Verification items for the finished model (mm, model axes). A direction names the side the tool comes from. Give positions to 0.01 mm unless a question says otherwise; leave off trailing zeros. Order: outer loops, then holes, each group sorted by start corner. A loop starts at its lowest first (then second) coordinate and runs counter-clockwise, first axis right, second up. Notation, with made-up numbers: M 5,-11 L 31,-11 A24 cw 31,12 Z; hole C 53,44.25 d7. An arc over 180 degrees is marked long. Answer as a JSON object with one key per item and string values.
```python
from build123d import *

# Parameters (mm, degrees)
F0_W      = 90
F0_H      = 90
F1_DEPTH  = 90
F2_W      = 30
F2_H      = 30
F3_DEPTH  = 30
F4_W      = 30
F4_H      = 30
F5_DEPTH  = 30
F6_W      = 30
F6_H      = 30
F7_DEPTH  = 30
F8_W      = 30
F8_H      = 30
F9_DEPTH  = 30
F10_W     = 30
F10_H     = 30
F11_DEPTH = 30
F12_W     = 30
F12_H     = 30
F13_DEPTH = 30


with BuildPart() as f1:
    # F0 (on Top) → F1 (new body)
    with BuildSketch(Plane.XY):
        Rectangle(F0_W, F0_H)
    extrude(amount=F1_DEPTH)

    # F2 (on face) → F3 (join)
    with BuildSketch(Plane(origin=(0, 0, 0), x_dir=(1, 0, 0), z_dir=(0, 0, -1))):
        with Locations((-30, 30)):
            Rectangle(F2_W, F2_H)
        with Locations((30, 30)):
            Rectangle(F2_W, F2_H)
        with Locations((-30, -30)):
            Rectangle(F2_W, F2_H)
        with Locations((30, -30)):
            Rectangle(F2_W, F2_H)
    extrude(amount=F3_DEPTH)

    # F4 (on face) → F5 (join)
    with BuildSketch(Plane(origin=(0, 45, 0), x_dir=(-1, 0, 0), z_dir=(0, 1, 0))):
        with Locations((30, 75)):
            Rectangle(F4_W, F4_H)
        with Locations((-30, 75)):
            Rectangle(F4_W, F4_H)
        with Locations((-30, 15)):
            Rectangle(F4_W, F4_H)
        with Locations((30, 15)):
            Rectangle(F4_W, F4_H)
    extrude(amount=F5_DEPTH)

    # F6 (on face) → F7 (join)
    with BuildSketch(Plane(origin=(-45, 0, 0), x_dir=(0, -1, 0), z_dir=(-1, 0, 0))):
        with Locations((-30, 75)):
            Rectangle(F6_W, F6_H)
        with Locations((-30, 15)):
            Rectangle(F6_W, F6_H)
        with Locations((30, 15)):
            Rectangle(F6_W, F6_H)
        with Locations((30, 75)):
            Rectangle(F6_W, F6_H)
    extrude(amount=F7_DEPTH)

    # F8 (on face) → F9 (join)
    with BuildSketch(Plane.YZ.offset(45)):
        with Locations((-30, 75)):
            Rectangle(F8_W, F8_H)
        with Locations((-30, 15)):
            Rectangle(F8_W, F8_H)
        with Locations((30, 15)):
            Rectangle(F8_W, F8_H)
        with Locations((30, 75)):
            Rectangle(F8_W, F8_H)
    extrude(amount=F9_DEPTH)

    # F10 (on face) → F11 (join)
    with BuildSketch(Plane.XZ.offset(45)):
        with Locations((-30, 75)):
            Rectangle(F10_W, F10_H)
        with Locations((-30, 15)):
            Rectangle(F10_W, F10_H)
        with Locations((30, 15)):
            Rectangle(F10_W, F10_H)
        with Locations((30, 75)):
            Rectangle(F10_W, F10_H)
    extrude(amount=F11_DEPTH)

    # F12 (on face) → F13 (join)
    with BuildSketch(Plane.XY.offset(90)):
        with Locations((-30, 30)):
            Rectangle(F12_W, F12_H)
        with Locations((-30, -30)):
            Rectangle(F12_W, F12_H)
        with Locations((30, -30)):
            Rectangle(F12_W, F12_H)
        with Locations((30, 30)):
            Rectangle(F12_W, F12_H)
    extrude(amount=F13_DEPTH)


solid = f1.part
```
Q1. Gauge pin test, flat ends, axial feed: pin 1 Ø24 at (y, z) = (-25, 100.5) entering from -X; pin 2 Ø12 at (x, y) = (-14, -57.5) entering from +Z; pin 3 Ø15 at (y, z) = (56, 68.5) entering from -X; pin 4 Ø10 at (x, z) = (27, 98) entering from -Y. Record the tip position at first contact, or that the pin passes through.
Resolved:
{"pin 1": "stops at x = -75", "pin 2": "stops at z = 90", "pin 3": "stops at x = -45", "pin 4": "stops at y = -45"}
Q2. Section check C-C on x = -34.5. Record the cut outline in (y, z), then the cut area to 3 significant figures.
Resolved:
{"outline": "M -75,0 L -45,0 L -45,-30 L -15,-30 L -15,0 L 15,0 L 15,-30 L 45,-30 L 45,0 L 75,0 L 75,30 L 45,30 L 45,60 L 75,60 L 75,90 L 45,90 L 45,120 L 15,120 L 15,90 L -15,90 L -15,120 L -45,120 L -45,90 L -75,90 L -75,60 L -45,60 L -45,30 L -75,30 Z", "area": "15,300 mm²"}
Q3. Section check B-B on y = 62.5. Record the cut outline in (x, z), then the cut area to 3 significant figures.
Resolved:
{"outline": "M -45,0 L -15,0 L -15,30 L -45,30 Z; M -45,60 L -15,60 L -15,90 L -45,90 Z; M 15,0 L 45,0 L 45,30 L 15,30 Z; M 15,60 L 45,60 L 45,90 L 15,90 Z", "area": "3,600 mm²"}
Q4. Material ranges on L1, parallel to Z at x = -65.5, y = 35; L2, parallel to X at y = -43.5, z = 105, recorded low to high.
Resolved:
{"L1": "z = 0 to 30, 60 to 90", "L2": "x = -45 to -15, 15 to 45"}
Q5. Release check for a two-part mould opening along X. For faces 1 (the face through (30, 30, 120)), 2 (the face through (-45, 60, 15)), 3 (the face through (-1, -45, 44)) record: +X half, -X half, draft (parallel to the pull), parting line (faces both ways), or undercut.
Resolved:
{"face 1": "draft", "face 2": "-X half", "face 3": "undercut"}
Q6. Tool access check on faces 4 (the face through (60, -45, 75)), 5 (the face through (15, -30, 105)), 6 (the face through (60, 45, 75)). Record the directions out of +Z, -Z, +X, -X, +Y, -Y that give a thin tool (end or side, any length) a straight path to the whole face; none if there is none.
Resolved:
{"face 4": "+Z, -Z, +X, -Y", "face 5": "+Z, +Y, -Y", "face 6": "+Z, -Z, +X, +Y"}
Q7. Section check A-A on z = 98. Record the cut outline in (x, y).
Resolved:
{"outline": "M -45,-45 L -15,-45 L -15,-15 L -45,-15 Z; M -45,15 L -15,15 L -15,45 L -45,45 Z; M 15,-45 L 45,-45 L 45,-15 L 15,-15 Z; M 15,15 L 45,15 L 45,45 L 15,45 Z"}
